Could you check a few things on this model? Use its own coordinates, in mm. Face numbers are marked on the shaded views. A direction names the side the tool comes from. Coordinates: 2 decimals unless noted, no trailing zeros. Loops run counter-clockwise (first coordinate to the right, second up) from the corner with the lowest first, then second, coordinate; pieces in that order, holes last. Notation, with made-up numbers: M 43.5,5 L 61.5,5 A24 cw 61.5,29 Z; hole C -7.5,49.25 d1. An arc over 180 degrees is marked long. Use one line per item in the form item = value. Start each with the question number.
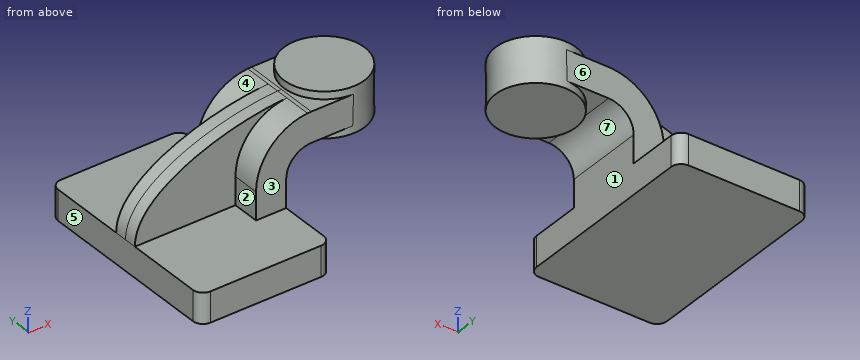
```python
from build123d import *

# Parameters (mm, degrees)
F1_DEPTH = 63.5
F0_W     = 25.3799454411
F0_H     = 19.05
F2_DEPTH = 25.4
F3_DEPTH = 7.9375
F5_R     = 6.35


with BuildPart() as f1:
    # F0 (on Front) → F1 (new body, symmetric)
    with BuildSketch(Plane.XZ):
        Polygon((41.275, -9.525), (41.275, 9.525), (22.225, 9.525), (-41.275, 9.525), (-41.275, -9.525), align=None)
    extrude(amount=F1_DEPTH, both=True)

    # F0 (on Front) → F2 (join, symmetric)
    with BuildSketch(Plane.XZ):
        with BuildLine():
            Line((22.225, 9.525), (41.275, 9.525))
            Line((41.275, 9.525), (41.275, 27.0002))
            ThreePointArc((41.275, 27.0002), (45.9246798487, 38.2255201513), (57.15, 42.8752))
            Line((57.15, 42.8752), (58.853423, 42.8752))
            Line((58.853423, 42.8752), (58.853423, 61.9252))
            Line((58.853423, 61.9252), (57.15, 61.9252))
            add(Edge.make_bspline(
                [(54.7810867094, 61.8447673645), (55.5787107168, 61.8791484879), (56.3685670715, 61.9059785826), (57.15, 61.9252)],
                knots=[109.2664103078, 109.2664103078, 109.2664103078, 109.2664103078, 111.5045361635, 111.5045361635, 111.5045361635, 111.5045361635], degree=3))
            ThreePointArc((54.7810867094, 61.8447673645), (31.6304984211, 50.8436616648), (22.225, 27.0002))
            Line((22.225, 27.0002), (22.225, 9.525))
        make_face()
        with Locations((71.5433957206, 52.4002)):
            Rectangle(F0_W, F0_H)
    extrude(amount=F2_DEPTH, both=True)

    # F0 (on Front) → F3 (join, symmetric)
    with BuildSketch(Plane.XZ):
        with BuildLine():
            Line((-41.275, 9.525), (22.225, 9.525))
            Line((22.225, 9.525), (22.225, 27.0002))
            ThreePointArc((22.225, 27.0002), (31.6304984211, 50.8436616648), (54.7810867094, 61.8447673645))
            add(Edge.make_bspline(
                [(-41.275, 9.525), (-41.6134486644, 40.4903317988), (15.8406885003, 60.1662639324), (54.7810867094, 61.8447673645)],
                knots=[0, 0, 0, 0, 109.2664103078, 109.2664103078, 109.2664103078, 109.2664103078], degree=3))
        make_face()
    extrude(amount=F3_DEPTH, both=True)

    # F0 (on Front) → F4 (revolve)
    with BuildSketch(Plane.XZ):
        Polygon((84.253423, 66.675), (84.2333684411, 38.1), (109.653423, 38.1), (109.653423, 66.675), align=None)
    revolve(axis=Axis((84.2433957206, 0, 52.3875), (-0.0007018217, 0, -0.9999997537)))

    # F5
    f5_edges = [f1.edges().sort_by_distance(p)[0] for p in [
        (41.275, -63.5, 0),
        (41.275, 63.5, 0),
        (-41.275, 63.5, 0),
        (-41.275, -63.5, 0),
    ]]
    fillet(f5_edges, radius=F5_R)


solid = f1.part
```
Item 1: Thinking about a two-plate mould opening in X: for the marked faces 5, 6 and 7, which applies, pulls with the +X half, pulls with the -X half, needs draft (parallel to the pull), parting line crosses it, or undercut?
Item 2: Please list where these lines run through material, in increasing order: line 1 along Y through (x, z) = (-3, 11); line 2 along Y through (x, z) = (26.5, 43); line 3 along X through (y, z) = (-47, 2.5) (3 decimals).
Item 3: I'm going to push flat-ended pins straight in: P1, Ø13.5, axis at x = 76.5, y = -11, coming from the +Z side; P2, Ø6, axis at y = 19.5, z = 36, coming from the +X side; P3, Ø4, axis at x = 36, y = 38.5, coming from the +Z side (3 decimals). Where does each tip first touch, or does it pass through?
Item 4: For the marked faces 1, 2, 3 and 4, which set-ups out of +Z, -Z, +X, -X, +Y, -Y let a thin tool reach every point of the face, with its end or its side?
Item 5: I want a section at A-A (z = -3.5). Write out the boundary of the cut face in (x, y) (3 decimals).
Item 6: I want a section at B-B (y = 34). Write out the boundary of the cut face in (x, z) (3 decimals).
Worked answers:
q1.face_5 = pulls with the -X half
q1.face_6 = needs draft
q1.face_7 = undercut
q2.line_1 = -7.94 to 7.94
q2.line_2 = -25.4 to 25.4
q2.line_3 = -41.275 to 41.275
q3.P1 = 66.7
q3.P2 = 102.8
q3.P3 = 9.525
q4.face_1 = -Z, +X, +Y, -Y
q4.face_2 = +Z, -X, -Y
q4.face_3 = +Z, +X, -X, -Y
q4.face_4 = +Z, -X, +Y
q5.outline = M -41.275,-57.15 A6.35 ccw -34.925,-63.5 L 34.925,-63.5 A6.35 ccw 41.275,-57.15 L 41.275,57.15 A6.35 ccw 34.925,63.5 L -34.925,63.5 A6.35 ccw -41.275,57.15 Z
q6.outline = M -41.275,-9.525 L 41.275,-9.525 L 41.275,9.525 L -41.275,9.525 Z
